Design review of the part built by this model. Coordinates are the model's own, in mm. A direction names the side the tool comes from. Coordinates: 2 decimals unless noted, no trailing zeros. Write each loop counter-clockwise with the first axis right and the second up, starting at its lowest first coordinate (ties: lowest second). Pieces come first, ordered by that corner, then holes.
Q1. The part is to be moulded in two halves that separate along Y. For faces 4 (the flat face through (11.5, -36, 3)), 5 (the cylindrical face through (-14.1, 7.57, 2.96)), 6 (the cylindrical face through (10.9, -12.43, 2.96)), 7 (the flat face through (0, -49, 3)), say which applies: released by +Y, released by -Y, zero draft, split by the parting line, or undercut.
Q2. Take a section at D-D, the plane y = 11. Write out the cut boundary in (x, z), plus the area to 3 significant figures.
Q3. Take a section at C-C, the plane x = 3. Write out the cut boundary in (y, z), plus the area to 3 significant figures.
Q4. For faces 1 (the flat face through (-11.5, -33, 3)), 2 (the flat face through (17.5, 6, 3)), 3 (the flat face through (4.5, -32, 3)), list the 3-axis set-ups (+Z, -Z, +X, -X, +Y, -Y) from which the entire face can be reached by the end or side of a thin tool; tool diameter is ignored.
Q5. Take a section at B-B, the plane x = 22. Write out the cut boundary in (y, z).
Q6. For L1, parallel to Y at x = 12.5, z = 1.4; L2, parallel to Y at x = -13, z = 4.15; L3, parallel to Y at x = 4, z = 1.7, list the stretches that pass through material, from the lowest coordinate up.
Q7. Take a section at A-A, the plane y = -12.5. Write out the cut boundary in (x, z).
Q8. For pin 1 Ø3 at (x, z) = (21, 3.5) entering from -Y; pin 2 Ø2.5 at (x, y) = (12.5, 7.5) entering from -Z; pin 3 Ø2 at (x, z) = (-7.5, 3) entering from -Y; pin 4 Ø0.9 at (y, z) = (-33, 3) entering from -X, all flat-tipped, find the tip position at first contact; note any pin that passes through.
from build123d import *

# Parameters (mm, degrees)
SKETCH1_R           = 1.6
SKETCH1_W           = 10
SKETCH1_H           = 12.4
SKETCH1_H_2         = 6.2
BOSS_EXTRUDE1_DEPTH = 6
SKETCH4_W           = 6
SKETCH4_H           = 20
BOSS_EXTRUDE2_DEPTH = 10
SKETCH7_W           = 6
SKETCH7_H           = 6
BOSS_EXTRUDE3_DEPTH = 16
CUT_EXTRUDE1_REACH  = 58.509
SKETCH6_W           = 6.2
SKETCH6_H           = 20
FILLET1_R           = 2
FILLET2_R           = 5


with BuildPart() as part:
    # Sketch1 → Boss-Extrude1 (new body)
    with BuildSketch(Plane.XY):
        Polygon((17.5, -20), (11.5, -20), (11.5, -49), (-11.5, -49), (-11.5, -20), (-17.5, -20), (-17.5, 15), (17.5, 15), align=None)
        with Locations((12.5, 7.5)):
            Circle(SKETCH1_R, mode=Mode.SUBTRACT)
        with Locations((-12.5, 7.5)):
            Circle(SKETCH1_R, mode=Mode.SUBTRACT)
        with Locations((-12.5, -12.5)):
            Circle(SKETCH1_R, mode=Mode.SUBTRACT)
        with Locations((12.5, -12.5)):
            Circle(SKETCH1_R, mode=Mode.SUBTRACT)
        with Locations((0, -12.5)):
            Rectangle(SKETCH1_W, SKETCH1_H, mode=Mode.SUBTRACT)
        with Locations((0, 9)):
            Rectangle(SKETCH1_W, SKETCH1_H_2, mode=Mode.SUBTRACT)
        with BuildLine():
            Line((-4.5, -33.8), (-4.5, -30.8))
            ThreePointArc((-4.5, -30.8), (0, -26.3), (4.5, -30.8))
            Line((4.5, -30.8), (4.5, -33.8))
            ThreePointArc((4.5, -33.8), (0, -38.3), (-4.5, -33.8))
        make_face(mode=Mode.SUBTRACT)
        with Locations((0, -44)):
            Rectangle(SKETCH1_W, SKETCH1_H_2, mode=Mode.SUBTRACT)
    extrude(amount=BOSS_EXTRUDE1_DEPTH)

    # Sketch4 → Boss-Extrude2 (add)
    with BuildSketch(Plane(origin=(17.5, 0, 0), x_dir=(0, 0, -1), z_dir=(1, 0, 0))):
        with Locations((-3, -10)):
            Rectangle(SKETCH4_W, SKETCH4_H)
    extrude(amount=BOSS_EXTRUDE2_DEPTH)

    # Sketch7 → Boss-Extrude3 (add)
    with BuildSketch(Plane(origin=(11.5, 0, 0), x_dir=(0, 0, -1), z_dir=(1, 0, 0))):
        with Locations((-3, -23)):
            Rectangle(SKETCH7_W, SKETCH7_H)
    extrude(amount=BOSS_EXTRUDE3_DEPTH)

    # Sketch6 → Cut-Extrude1 (cut, up to next)
    with BuildSketch(Plane.XY.offset(6), mode=Mode.PRIVATE) as cut_extrude1_sk1:
        with Locations((20.5, -13)):
            Rectangle(SKETCH6_W, SKETCH6_H)
    cut_extrude1_tool1 = extrude(cut_extrude1_sk1.sketch, amount=-CUT_EXTRUDE1_REACH, mode=Mode.PRIVATE) & part.part
    add(cut_extrude1_tool1.solids().sort_by_distance((20.5, -13, 6))[0], mode=Mode.SUBTRACT)

    # Fillet1
    fillet1_edges = [part.edges().sort_by_distance(p)[0] for p in [
        (27.5, 0, 3),
        (11.5, -26, 3),
        (27.5, -26, 3),
        (-11.5, -20, 3),
        (-17.5, -20, 3),
        (17.5, 0, 3),
    ]]
    fillet(fillet1_edges, radius=FILLET1_R)

    # Fillet2
    fillet2_edges = [part.edges().sort_by_distance(p)[0] for p in [
        (-17.5, 15, 3),
        (17.5, 15, 3),
        (11.5, -49, 3),
        (-11.5, -49, 3),
    ]]
    fillet(fillet2_edges, radius=FILLET2_R)


solid = part.part
Responses:
1. face 4: zero draft
1. face 5: undercut
1. face 6: undercut
1. face 7: released by -Y
2. outline: (-17.4, 0) - (-5, 0) - (-5, 6) - (-17.4, 6) - close; (5, 0) - (17.4, 0) - (17.4, 6) - (5, 6) - close
2. area: 149 mm2
3. outline: (-49, 0) - (-47.1, 0) - (-47.1, 6) - (-49, 6) - close; (-40.9, 0) - (-37.15, 0) - (-37.15, 6) - (-40.9, 6) - close; (-27.45, 0) - (-18.7, 0) - (-18.7, 6) - (-27.45, 6) - close; (-6.3, 0) - (5.9, 0) - (5.9, 6) - (-6.3, 6) - close; (12.1, 0) - (15, 0) - (15, 6) - (12.1, 6) - close
3. area: 177 mm2
4. face 1: +Z, -Z, -X, -Y
4. face 2: +Z, -Z, +X, +Y
4. face 3: +Z, -Z
5. outline: (-26, 0) - (-23, 0) - (-23, 6) - (-26, 6) - close; (-3, 0) - (0, 0) - (0, 6) - (-3, 6) - close
6. L1: y = -26.27 to -14.1, -10.9 to 5.9, 9.1 to 15
6. L2: y = -20.06 to -14.02, -10.98 to 5.98, 9.02 to 14.97
6. L3: y = -49 to -47.1, -40.9 to -35.86, -28.74 to -18.7, -6.3 to 5.9, 12.1 to 15
7. outline: (-17.5, 0) - (-14.1, 0) - (-14.1, 6) - (-17.5, 6) - close; (-10.9, 0) - (-5, 0) - (-5, 6) - (-10.9, 6) - close; (5, 0) - (10.9, 0) - (10.9, 6) - (5, 6) - close; (14.1, 0) - (17.4, 0) - (17.4, 6) - (14.1, 6) - close; (23.6, 0) - (27.5, 0) - (27.5, 6) - (23.6, 6) - close
8. pin 1: stops at y = -26
8. pin 2: passes through
8. pin 3: stops at y = -49
8. pin 4: stops at x = -11.5
